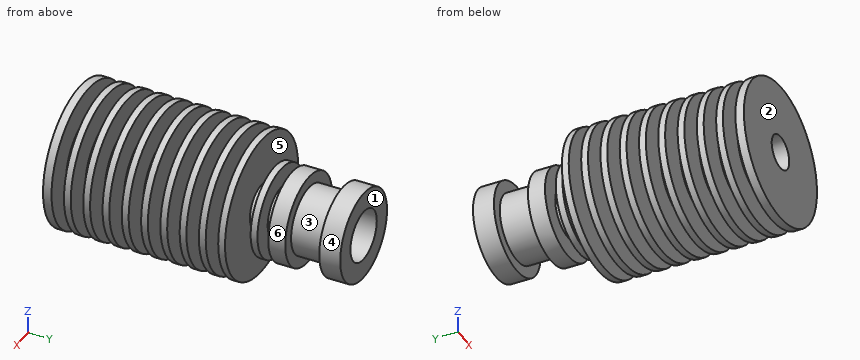
from build123d import *


with BuildPart() as part:
    # Skica1 → Rotovat1 (revolve)
    with BuildSketch(Plane.XY, mode=Mode.PRIVATE) as rotovat1_sk:
        Polygon((8, 64.637455621), (4.5, 64.637455621), (4.5, 52.97460351), (2, 50.637455621), (2, 46.936179321), (1, 46.637455621), (1, 33.037455621), (1, 31.837455621), (3, 31.837455621), (3, 14.537455621), (12.5, 14.537455621), (12.5, 16.037455621), (7.5, 16.037455621), (7.5, 18.237455621), (12.5, 18.237455621), (12.5, 19.437455621), (7.5, 19.437455621), (7.5, 21.637455621), (12.5, 21.637455621), (12.5, 22.837455621), (7.5, 22.837455621), (7.5, 25.037455621), (12.5, 25.037455621), (12.5, 26.237455621), (7.5, 26.237455621), (7.5, 28.437455621), (12.5, 28.437455621), (12.5, 29.637455621), (7.5, 29.637455621), (7.5, 31.837455621), (12.5, 31.837455621), (12.5, 33.037455621), (6.5, 33.037455621), (6.5, 35.237455621), (12.5, 35.237455621), (12.5, 36.437455621), (4, 36.437455621), (4, 38.637455621), (12.5, 38.637455621), (12.5, 39.837455621), (4, 39.837455621), (4, 42.037455621), (12.5, 42.037455621), (12.5, 43.237455621), (4, 43.237455621), (4, 45.437455621), (12.5, 45.437455621), (12.5, 46.637455621), (4, 46.637455621), (4, 48.837455621), (8, 48.837455621), (8, 50.037455621), (4.5, 50.037455621), (4.5, 51.937455621), (8, 51.937455621), (8, 54.937455621), (6, 54.937455621), (6, 60.937455621), (8, 60.937455621), align=None)
    revolve(rotovat1_sk.sketch.rotate(Axis((0, 64.637455621, 0), (0, -1, 0)), 180), axis=Axis((0, 64.637455621, 0), (0, -1, 0)))


solid = part.part
Build history of the part. All positions in model axes, mm. Face numbers are marked on the shaded views. A direction names the side the tool comes from. Coordinates: 2 decimals unless noted, no trailing zeros. Write each loop counter-clockwise with the first axis right and the second up, starting at its lowest first coordinate (ties: lowest second). Pieces come first, ordered by that corner, then holes.
(1) Pin check, flat tips, straight feed: pin 1 Ø12.5 at (x, z) = (1.5, -2) entering from +Y; pin 2 Ø7 at (x, z) = (0, 0) entering from +Y; pin 3 Ø1 at (y, z) = (30, 7.5) entering from -X; pin 4 Ø8 at (x, z) = (8.5, 9) entering from +Y. Stop position of each tip, or through.
(2) Cut at D-D on y = 30.5. List the corners of the cut face in (x, z).
(3) Cut at A-A on z = 10. State how many separate pieces and enclosed holes the cut face has, and give its area (4 significant figures).
(4) Cut at B-B on y = 55.5. List the corners of the cut face in (x, z), and give its area (3 significant figures).
(5) 3-axis set-ups, long thin cutter, end or side, ignore diameter. For the marked faces 5 and 6: which of +Z, -Z, +X, -X, +Y, -Y reach the whole face in a straight line?
(6) Mould opens along Y. For the marked faces 1, 2, 3 and 4 say: pulls with the +Y half, pulls with the -Y half, needs draft (parallel to the pull), parting line crosses it, or undercut.
(7) Drill centre lines: line 1 (Z direction, x = 0, y = 48.95); line 2 (Y direction, x = -1, z = 4.25); line 3 (Z direction, x = 0, y = 48.55). Where is each one in solid material? Low to high.
Working result:
1. pin 1: stops at y = 64.64
1. pin 2: stops at y = 52.04
1. pin 3: stops at x = -10.25
1. pin 4: stops at y = 46.64
2. outline: circle Ø15 at (0, 0); hole circle Ø6 at (0, 0)
3. separate pieces: 10
3. enclosed holes: 0
3. area: 184.5 mm2
4. outline: circle Ø12 at (0, 0); hole circle Ø9 at (0, 0)
4. area: 49.5 mm2
5. face 5: none
5. face 6: +Y
6. face 1: pulls with the +Y half
6. face 2: pulls with the -Y half
6. face 3: undercut
6. face 4: needs draft
7. line 1: z = -8 to -2, 2 to 8
7. line 2: y = 14.54 to 36.44, 38.64 to 39.84, 42.04 to 43.24, 45.44 to 46.64, 48.84 to 52.85
7. line 3: z = -4 to -2, 2 to 4
